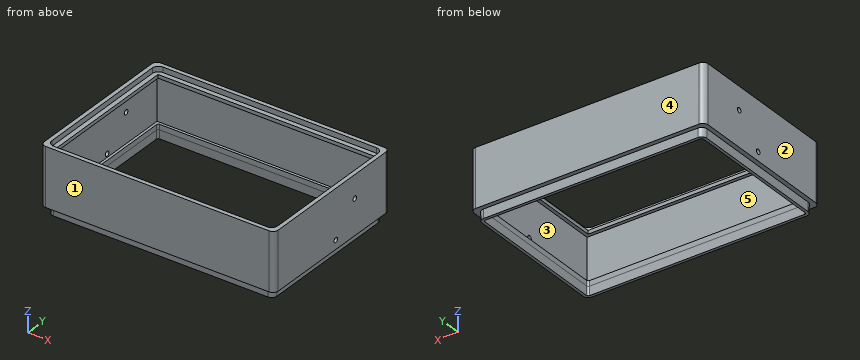
Autodesk Inventor part; units mm, degrees
ref_plane "Arbeitsebene3" through (-63.945, -42.8, 0) normal (0, 0, 1) x (1, 0, 0)
ref_plane "YZ Plane" through (0, 0, 0) normal (1, 0, 0) x (0, 1, 0)
ref_plane "XZ Plane" through (0, 0, 0) normal (0, 1, 0) x (-1, 0, 0)
ref_plane "Arbeitsebene1" through (0, 0, 0) normal (0, 0, 1) x (1, 0, 0)
ref_plane "Arbeitsebene2" through (0, 0, 5) normal (0, 0, 1) x (1, 0, 0)
sketch "Skizze2" plane through (0, 0, 5) normal (0, 0, 1) x (1, 0, 0)
  arc A0 (-24.056, -76.2783) -> (-18.8, -75.35) centre (-21.51, -75.35) ccw
  arc A1 (63.445, -45.3) -> (66.445, -42.3) centre (63.445, -42.3) ccw
  line L0 (66.445, -42.3) -> (66.445, 42.3)
  arc A2 (66.445, 42.3) -> (63.445, 45.3) centre (63.445, 42.3) ccw
  line L1 (63.445, 45.3) -> (-63.445, 45.3)
  arc A3 (-63.445, 45.3) -> (-66.445, 42.3) centre (-63.445, 42.3) ccw
  line L2 (-66.445, 42.3) -> (-66.445, -42.3)
  arc A4 (-66.445, -42.3) -> (-63.445, -45.3) centre (-63.445, -42.3) ccw
  line L3 (-63.445, -45.3) -> (63.445, -45.3)
  arc A5 (63.945, 39.8) -> (60.945, 42.8) centre (60.945, 39.8) ccw
  line L4 (63.945, 39.8) -> (63.945, -39.8)
  arc A6 (60.945, -42.8) -> (63.945, -39.8) centre (60.945, -39.8) ccw
  line L5 (60.945, -42.8) -> (-60.945, -42.8)
  arc A7 (-63.945, -39.8) -> (-60.945, -42.8) centre (-60.945, -39.8) ccw
  line L6 (-63.945, -39.8) -> (-63.945, 39.8)
  arc A8 (-60.945, 42.8) -> (-63.945, 39.8) centre (-60.945, 39.8) ccw
  line L7 (-60.945, 42.8) -> (60.945, 42.8)
  line L8 (-61.945, 39.8) -> (-61.945, -39.8)
  arc A9 (-61.945, -39.8) -> (-60.945, -40.8) centre (-60.945, -39.8) ccw
  line L9 (-60.945, -40.8) -> (60.945, -40.8)
  arc A10 (60.945, -40.8) -> (61.945, -39.8) centre (60.945, -39.8) ccw
  line L10 (61.945, -39.8) -> (61.945, 39.8)
  arc A11 (61.945, 39.8) -> (60.945, 40.8) centre (60.945, 39.8) ccw
  line L11 (60.945, 40.8) -> (-60.945, 40.8)
  arc A12 (-60.945, 40.8) -> (-61.945, 39.8) centre (-60.945, 39.8) ccw
  point P0 (0, 0)
  dimension "d1" = 2
ref_plane "Arbeitsebene3" through (-63.945, -42.8, 0) normal (0, 0, 1) x (1, 0, 0)
extrude "Extrusion1" add sketch "Skizze2" against normal up to surface (5 mm away) draft -2 contours L4 A6 L5 A7 L6 A8 L7 A5
sketch "Skizze3" plane through (0, 0, 5) normal (0, 0, 1) x (1, 0, 0)
  arc A0 (63.445, -45.3) -> (66.445, -42.3) centre (63.445, -42.3) ccw
  line L0 (66.445, -42.3) -> (66.445, 42.3)
  arc A1 (66.445, 42.3) -> (63.445, 45.3) centre (63.445, 42.3) ccw
  line L1 (63.445, 45.3) -> (-63.445, 45.3)
  arc A2 (-63.445, 45.3) -> (-66.445, 42.3) centre (-63.445, 42.3) ccw
  line L2 (-66.445, 42.3) -> (-66.445, -42.3)
  arc A3 (-66.445, -42.3) -> (-63.445, -45.3) centre (-63.445, -42.3) ccw
  line L3 (-63.445, -45.3) -> (63.445, -45.3)
  arc A4 (63.945, 39.8) -> (60.945, 42.8) centre (60.945, 39.8) ccw
  line L4 (63.945, 39.8) -> (63.945, -39.8)
  arc A5 (60.945, -42.8) -> (63.945, -39.8) centre (60.945, -39.8) ccw
  line L5 (60.945, -42.8) -> (-60.945, -42.8)
  arc A6 (-63.945, -39.8) -> (-60.945, -42.8) centre (-60.945, -39.8) ccw
  line L6 (-63.945, -39.8) -> (-63.945, 39.8)
  arc A7 (-60.945, 42.8) -> (-63.945, 39.8) centre (-60.945, 39.8) ccw
  line L7 (-60.945, 42.8) -> (60.945, 42.8)
  line L8 (-61.945, -39.8) -> (-61.945, 39.8)
  arc A8 (-60.945, 40.8) -> (-61.945, 39.8) centre (-60.945, 39.8) ccw
  line L9 (-60.945, 40.8) -> (60.945, 40.8)
  arc A9 (61.945, 39.8) -> (60.945, 40.8) centre (60.945, 39.8) ccw
  line L10 (61.945, 39.8) -> (61.945, -39.8)
  arc A10 (60.945, -40.8) -> (61.945, -39.8) centre (60.945, -39.8) ccw
  line L11 (60.945, -40.8) -> (-60.945, -40.8)
  arc A11 (-61.945, -39.8) -> (-60.945, -40.8) centre (-60.945, -39.8) ccw
  line L12 (63.945, -39.8) -> (63.945, 39.8)
  arc A12 (63.945, 39.8) -> (60.945, 42.8) centre (60.945, 39.8) ccw
  line L13 (60.945, 42.8) -> (-60.945, 42.8)
  arc A13 (-60.945, 42.8) -> (-63.945, 39.8) centre (-60.945, 39.8) ccw
  line L14 (-63.945, 39.8) -> (-63.945, -39.8)
  arc A14 (-63.945, -39.8) -> (-60.945, -42.8) centre (-60.945, -39.8) ccw
  line L15 (-60.945, -42.8) -> (60.945, -42.8)
  arc A15 (60.945, -42.8) -> (63.945, -39.8) centre (60.945, -39.8) ccw
  point P0 (0, 0)
extrude "Extrusion2" add sketch "Skizze3" along normal blind 3 contours L3 A3 L2 A2 L1 A1 L0 A0 | L4 A5 L5 A6 L6 A7 L7 A4
sketch "Skizze4" plane through (0, 0, 8) normal (0, 0, 1) x (1, 0, 0)
  line L0 (66.445, -42.3) -> (66.445, 42.3)
  arc A0 (66.445, 42.3) -> (63.445, 45.3) centre (63.445, 42.3) ccw
  line L1 (63.445, 45.3) -> (-63.445, 45.3)
  arc A1 (-63.445, 45.3) -> (-66.445, 42.3) centre (-63.445, 42.3) ccw
  line L2 (-66.445, 42.3) -> (-66.445, -42.3)
  arc A2 (-66.445, -42.3) -> (-63.445, -45.3) centre (-63.445, -42.3) ccw
  line L3 (-63.445, -45.3) -> (63.445, -45.3)
  arc A3 (63.445, -45.3) -> (66.445, -42.3) centre (63.445, -42.3) ccw
  line L4 (60.945, -40.8) -> (-60.945, -40.8)
  arc A4 (-61.945, -39.8) -> (-60.945, -40.8) centre (-60.945, -39.8) ccw
  line L5 (-61.945, -39.8) -> (-61.945, 39.8)
  arc A5 (-60.945, 40.8) -> (-61.945, 39.8) centre (-60.945, 39.8) ccw
  line L6 (-60.945, 40.8) -> (60.945, 40.8)
  arc A6 (61.945, 39.8) -> (60.945, 40.8) centre (60.945, 39.8) ccw
  line L7 (61.945, 39.8) -> (61.945, -39.8)
  arc A7 (60.945, -40.8) -> (61.945, -39.8) centre (60.945, -39.8) ccw
  line L8 (-63.445, -42.3) -> (-63.445, 42.3)
  line L9 (-63.445, 42.3) -> (63.445, 42.3)
  line L10 (63.445, 42.3) -> (63.445, -42.3)
  line L11 (63.445, -42.3) -> (-63.445, -42.3)
  point P0 (0, 0)
  dimension "d6" = 3
extrude "Extrusion3" add sketch "Skizze4" along normal blind 25 contours A3 L3 A2 L2 A1 L1 A0 L0
sketch "Skizze5" plane through (0, 0, 33) normal (0, 0, 1) x (1, 0, 0)
  arc A0 (66.445, 42.3) -> (63.445, 45.3) centre (63.445, 42.3) ccw
  line L0 (63.445, 45.3) -> (-63.445, 45.3)
  arc A1 (-63.445, 45.3) -> (-66.445, 42.3) centre (-63.445, 42.3) ccw
  line L1 (-66.445, 42.3) -> (-66.445, -42.3)
  arc A2 (-66.445, -42.3) -> (-63.445, -45.3) centre (-63.445, -42.3) ccw
  line L2 (-63.445, -45.3) -> (63.445, -45.3)
  arc A3 (63.445, -45.3) -> (66.445, -42.3) centre (63.445, -42.3) ccw
  line L3 (66.445, -42.3) -> (66.445, 42.3)
  line L4 (-63.445, -42.3) -> (-63.445, 42.3)
  line L5 (-63.445, 42.3) -> (63.445, 42.3)
  line L6 (63.445, 42.3) -> (63.445, -42.3)
  line L7 (63.445, -42.3) -> (-63.445, -42.3)
  line L8 (-61.445, -40.3) -> (-61.445, 40.3)
  line L9 (-61.445, 40.3) -> (61.445, 40.3)
  line L10 (61.445, 40.3) -> (61.445, -40.3)
  line L11 (61.445, -40.3) -> (-61.445, -40.3)
  point P0 (0, 0)
  dimension "d9" = 2
extrude "Extrusion4" add sketch "Skizze5" along normal blind 2 contours L3 A3 L2 A2 L1 A1 L0 A0 | L4 L5 L6 L7
sketch "Skizze6" plane through (0, 0, 35) normal (0, 0, 1) x (1, 0, 0)
  line L0 (-60.625, -42.48) -> (60.625, -42.48)
  arc A0 (-63.625, -39.48) -> (-60.625, -42.48) centre (-60.625, -39.48) ccw
  line L1 (-63.625, 39.48) -> (-63.625, -39.48)
  arc A1 (-60.625, 42.48) -> (-63.625, 39.48) centre (-60.625, 39.48) ccw
  line L2 (60.625, 42.48) -> (-60.625, 42.48)
  arc A2 (63.625, 39.48) -> (60.625, 42.48) centre (60.625, 39.48) ccw
  line L3 (63.625, -39.48) -> (63.625, 39.48)
  arc A3 (60.625, -42.48) -> (63.625, -39.48) centre (60.625, -39.48) ccw
  line L4 (53.1911, 40.1013) -> (61.2463, 32.0461)
  arc A4 (53.1911, 40.1013) -> (51.0698, 40.98) centre (51.0698, 37.98) ccw
  line L5 (51.0698, 40.98) -> (-59.125, 40.98)
  arc A5 (-59.125, 40.98) -> (-62.125, 37.98) centre (-59.125, 37.98) ccw
  line L6 (-62.125, 37.98) -> (-62.125, -37.98)
  arc A6 (-62.125, -37.98) -> (-59.125, -40.98) centre (-59.125, -37.98) ccw
  line L7 (-59.125, -40.98) -> (51.0698, -40.98)
  arc A7 (51.0698, -40.98) -> (53.1911, -40.1013) centre (51.0698, -37.98) ccw
  line L8 (61.2463, -32.0461) -> (53.1911, -40.1013)
  arc A8 (61.2463, -32.0461) -> (62.125, -29.9248) centre (59.125, -29.9248) ccw
  line L9 (62.125, -29.9248) -> (62.125, 29.9248)
  arc A9 (62.125, 29.9248) -> (61.2463, 32.0461) centre (59.125, 29.9248) ccw
  arc A10 (-64.125, -39.48) -> (-60.625, -42.98) centre (-60.625, -39.48) ccw
  line L10 (-60.625, -42.98) -> (60.625, -42.98)
  arc A11 (60.625, -42.98) -> (64.125, -39.48) centre (60.625, -39.48) ccw
  line L11 (64.125, -39.48) -> (64.125, 39.48)
  arc A12 (64.125, 39.48) -> (60.625, 42.98) centre (60.625, 39.48) ccw
  line L12 (60.625, 42.98) -> (-60.625, 42.98)
  arc A13 (-60.625, 42.98) -> (-64.125, 39.48) centre (-60.625, 39.48) ccw
  line L13 (-64.125, 39.48) -> (-64.125, -39.48)
  line L14 (63.445, 45.3) -> (-63.445, 45.3)
  arc A14 (-63.445, 45.3) -> (-66.445, 42.3) centre (-63.445, 42.3) ccw
  line L15 (-66.445, 42.3) -> (-66.445, -42.3)
  arc A15 (-66.445, -42.3) -> (-63.445, -45.3) centre (-63.445, -42.3) ccw
  line L16 (-63.445, -45.3) -> (63.445, -45.3)
  arc A16 (63.445, -45.3) -> (66.445, -42.3) centre (63.445, -42.3) ccw
  line L17 (66.445, -42.3) -> (66.445, 42.3)
  arc A17 (66.445, 42.3) -> (63.445, 45.3) centre (63.445, 42.3) ccw
  line L18 (-61.445, -40.3) -> (-61.445, 40.3)
  line L19 (-61.445, 40.3) -> (61.445, 40.3)
  line L20 (61.445, 40.3) -> (61.445, -40.3)
  line L21 (61.445, -40.3) -> (-61.445, -40.3)
  point P0 (0, 0)
  dimension "d12" = 0.5
extrude "Extrusion5" add sketch "Skizze6" along normal blind 3 contours A17 L17 A16 L16 A15 L15 A14 L14
sketch "Skizze7" plane through (66.445, -42.3, 5) normal (1, 0, 0) x (0, 0, -1)
  circle A0 centre (-5.052, 45.2732) radius 1.49
  circle A1 centre (-20.052, 60.2732) radius 1.4
  point P0 (5, 42.3)
hole "Bohrung1" at (66.445, 2.9732, 10.052) at (66.445, 17.9732, 25.052) direction (-1, 0, 0) diameter 2.8 end through all
properties part number "NematostellaImager_spacer_v0"
Input: part model. Units: mm. Frame: model coordinates. Face numbers are marked on the shaded views. A direction names the side the tool comes from. Give positions to 0.01 mm unless a question says otherwise; leave off trailing zeros. Loops run counter-clockwise (first coordinate to the right, second up) from the corner with the lowest first, then second, coordinate; pieces in that order, holes last. Notation, with made-up numbers: (0, 11.5) -> (41, 11.5) arc R22 ccw to (41, 45.5) -> close; hole circle Ø11 at (-32.5, 76). An arc over 180 degrees is marked (long way). Answer as a JSON object with one key per item and string values. Group by question number.
Item 1: Cut plane C-C, the plane z = 21.5. Return the cut outline in (x, y) (3 decimals), and give its area (3 significant figures).
Item 2: Cut plane B-B, the plane x = 3. Return the cut outline in (y, z), and give its area (3 significant figures).
Item 3: Reachability of the marked faces 4 and 5 from +Z, -Z, +X, -X, +Y, -Y: full face, straight path, thin tool, end or side. Return the list, or none.
Item 4: Line query: probe 1 along X at (y, z) = (9, 24) (3 decimals); probe 2 along X at (y, z) = (32, 36) (3 decimals); probe 3 along Y at (x, z) = (29, 10). Output: solid intervals per line, ascending.
Item 5: Pull-direction query (X, two-part tool) for the marked faces 1, 2 and 3; classes: released by +X, released by -X, zero draft, split by the parting line, or undercut.
Item 6: Cut plane A-A, the plane y = 6. Return the cut outline in (x, z) (3 decimals).
Checks:
{
 "1": {"outline": "(-66.445, -42.3) arc R3 ccw to (-63.445, -45.3) -> (63.445, -45.3) arc R3 ccw to (66.445, -42.3) -> (66.445, 42.3) arc R3 ccw to (63.445, 45.3) -> (-63.445, 45.3) arc R3 ccw to (-66.445, 42.3) -> close; hole (-63.445, -42.3) -> (63.445, -42.3) -> (63.445, 42.3) -> (-63.445, 42.3) -> close", "area": "1,300 mm²"},
 "2": {"outline": "(-45.3, 5) -> (-42.8, 5) -> (-42.63, 0) -> (-40.97, 0) -> (-40.8, 5) -> (-40.8, 8) -> (-42.3, 8) -> (-42.3, 33) -> (-40.3, 33) -> (-40.3, 35) -> (-42.98, 35) -> (-42.98, 38) -> (-45.3, 38) -> close; (40.3, 33) -> (42.3, 33) -> (42.3, 8) -> (40.8, 8) -> (40.8, 5) -> (40.97, 0) -> (42.63, 0) -> (42.8, 5) -> (45.3, 5) -> (45.3, 38) -> (42.98, 38) -> (42.98, 35) -> (40.3, 35) -> close", "area": "229 mm²"},
 "3": {"face 4": "+Z, -Z, +X, -X, +Y", "face 5": "none"},
 "4": {"probe 1": "x = -66.445 to -63.445, 63.445 to 66.445", "probe 2": "x = -66.445 to -64.125, 64.125 to 66.445", "probe 3": "y = -45.3 to -42.3, 42.3 to 45.3"},
 "5": {"face 1": "zero draft", "face 2": "released by -X", "face 3": "undercut"},
 "6": {"outline": "(-66.445, 5) -> (-63.945, 5) -> (-63.77, 0) -> (-62.12, 0) -> (-61.945, 5) -> (-61.945, 8) -> (-63.445, 8) -> (-63.445, 33) -> (-61.445, 33) -> (-61.445, 35) -> (-64.125, 35) -> (-64.125, 38) -> (-66.445, 38) -> close; (61.445, 33) -> (63.445, 33) -> (63.445, 8) -> (61.945, 8) -> (61.945, 5) -> (62.12, 0) -> (63.77, 0) -> (63.945, 5) -> (66.445, 5) -> (66.445, 38) -> (64.125, 38) -> (64.125, 35) -> (61.445, 35) -> close"}
}
